Work out the finished part from the listing and answer in its coordinate system (mm). Face numbers are marked on the shaded views. Coordinates: 2 decimals unless noted, no trailing zeros. Write each loop counter-clockwise with the first axis right and the second up, starting at its lowest first coordinate (ties: lowest second). Pieces come first, ordered by that corner, then holes. Notation, with made-up numbers: M -35,-21.5 L -5,-21.5 A19 ccw -5,-16.5 Z; hole C 9,33.5 d2. An arc over 180 degrees is marked long. Use CSV: the item, a comma, the result in double quotes.
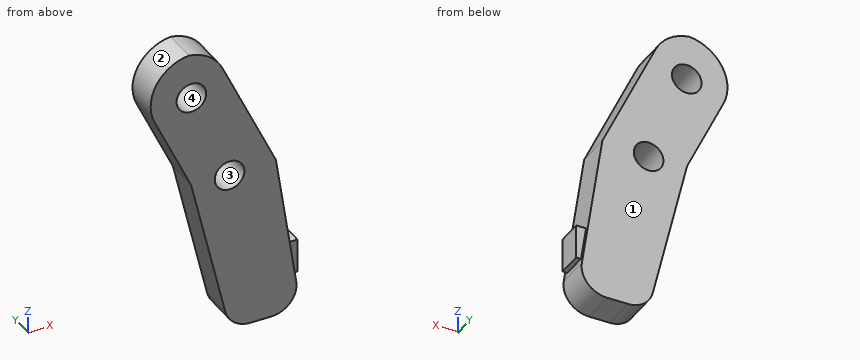
from build123d import *

# Parameters (mm, degrees)
BOSS_EXTRUDE1_DEPTH = 4
FILLET1_R           = 5
FILLET2_R           = 3
SKETCH2_R           = 1.75
CUT_EXTRUDE1_DEPTH  = 42.213228115
BOSS_EXTRUDE2_REACH = 42.084
SKETCH4_W           = 4
SKETCH4_H           = 3


with BuildPart() as part:
    # Sketch1 → Boss-Extrude1 (new body)
    with BuildSketch(Plane(origin=(0, 0, 0), x_dir=(1, 0, 0), z_dir=(0, 1, 0))):
        Polygon((0, 0), (7.627319971, 16.304109607), (12.214275277, 35.771000499), (20.559764671, 35.771000499), (17.627319971, 16.304109607), (10, 0), align=None)
    extrude(amount=BOSS_EXTRUDE1_DEPTH)

    # Fillet1
    # the kernel refuses this fillet: 5 mm, written as the material it takes off along each edge
    with BuildSketch(Plane(origin=(10, -7.952504215, 0), x_dir=(0.42373999836860227, 0, -0.9057838670359375), z_dir=(0, 1, 0))) as fillet1_piece_1:
        with BuildLine():
            CenterArc((FILLET1_R * 0.636200337192, FILLET1_R), FILLET1_R, 205.070935448, 64.929064552)
            Line((-FILLET1_R * 0.269583529844, FILLET1_R * 0.576260001631), (0, 0))
            Line((0, 0), (FILLET1_R * 0.636200337192, 0))
        make_face()
    extrude(amount=19.90500843, mode=Mode.SUBTRACT)
    with BuildSketch(Plane(origin=(0, -19.647899049, 0), x_dir=(0.42373999836860193, 0, -0.9057838670359376), z_dir=(0, 1, 0))) as fillet1_piece_2:
        with BuildLine():
            CenterArc((FILLET1_R * 1.57183192391, -FILLET1_R), FILLET1_R, 90, 115.070935448)
            Line((FILLET1_R * 0.666048056873, -FILLET1_R * 1.42373999837), (0, 0))
            Line((0, 0), (FILLET1_R * 1.57183192391, 0))
        make_face()
    extrude(amount=43.295798098, mode=Mode.SUBTRACT)

    # Fillet2
    fillet2_edges = [part.edges().sort_by_distance(p)[0] for p in [
        (12.214275277, 2, -35.771000499),
        (20.559764671, 2, -35.771000499),
    ]]
    fillet(fillet2_edges, radius=FILLET2_R)

    # Sketch2 → Cut-Extrude1 (cut, through all)
    with BuildSketch(Plane(origin=(0, 4, 0), x_dir=(1, 0, 0), z_dir=(0, 1, 0))):
        with Locations(Location((7.667711585, 5.413915862, 0), (0, 0, 270))):
            Circle(SKETCH2_R)
        with Locations(Location((12.170024678, 16.537277621, 0), (0, 0, 270))):
            Circle(SKETCH2_R)
    extrude(amount=-CUT_EXTRUDE1_DEPTH, mode=Mode.SUBTRACT)

    # Boss-Extrude2: up to this plane
    boss_extrude2_end = Plane(origin=(17.627319971, 4, -16.304109607), z_dir=(-0.9888436763539994, 0, -0.1489569861896618))
    # Sketch4 → Boss-Extrude2 (add, up to the surface)
    with BuildSketch(Plane(origin=(20.5, 0, 0), x_dir=(0, 0, -1), z_dir=(1, 0, 0)), mode=Mode.PRIVATE) as boss_extrude2_sk1:
        with Locations((29.561107497, 2.091926215)):
            Rectangle(SKETCH4_W, SKETCH4_H)
    boss_extrude2_tool1 = split(extrude(boss_extrude2_sk1.sketch, amount=-BOSS_EXTRUDE2_REACH, mode=Mode.PRIVATE), bisect_by=boss_extrude2_end, keep=Keep.BOTH, mode=Mode.PRIVATE)
    add(boss_extrude2_tool1.solids().sort_by_distance((20.5, 2.091926, -29.561107))[0])


solid = part.part
Item 1: Consider probe 1 along X at (y, z) = (1.65, -6); probe 2 along X at (y, z) = (1.85, -18); probe 3 along Z at (x, y) = (6.75, 1.6). Determine where each line is inside the solid, lowest interval first.
Answer:
probe 1,"x = 2.96 to 6.02, 9.32 to 12.81"
probe 2,"x = 8.03 to 11.21, 13.13 to 17.88"
probe 3,"z = -14.43 to -6.9, -3.92 to -0.12"
Item 2: The part is cut by section A-A (x = 7). Write down the section's boundary in (y, z), then the cut area to 3 significant figures.
Answer:
outline,"M 0,-14.96 L 4,-14.96 L 4,-7.03 L 0,-7.03 Z; M 0,-3.8 L 4,-3.8 L 4,-0.07 L 0,-0.07 Z"
area,"46.6 mm2"
Item 3: The part is cut by section B-B (y = 2.3). Write down the section's boundary in (x, z), then the cut area to 3 significant figures.
Answer:
outline,"M 3.33,-7.12 L 7.63,-16.3 L 11.67,-33.46 A3 ccw 14.59,-35.77 L 17.07,-35.77 A3 ccw 20.04,-32.32 L 19.93,-31.56 L 20.5,-31.56 L 20.5,-27.56 L 19.32,-27.56 L 17.63,-16.3 L 11.35,-2.88 A5 ccw 7.34,-0.03 A5 ccw Z; hole C 7.67,-5.41 d3.5; hole C 12.17,-16.54 d3.5"
area,"306 mm2"
Item 4: The part is cut by section C-C (z = -31). Write down the section's boundary in (x, y), then the cut area to 3 significant figures.
Answer:
outline,"M 11.09,0 L 19.84,0 L 19.84,0.59 L 20.5,0.59 L 20.5,3.59 L 19.84,3.59 L 19.84,4 L 11.09,4 Z"
area,"37.0 mm2"
Item 5: For a pull along Z with two mould halves and no side action, classify the marked faces 1, 2, 3 and 4 as released by +Z, released by -Z, zero draft, split by the parting line, or undercut.
Answer:
face 1,"zero draft"
face 2,"split by the parting line"
face 3,"undercut"
face 4,"undercut"
Item 6: The part is cut by section D-D (x = 12.5). Write down the section's boundary in (y, z).
Answer:
outline,"M 0,-34.92 L 4,-34.92 L 4,-18.26 L 0,-18.26 Z; M 0,-14.82 L 4,-14.82 L 4,-5.34 L 0,-5.34 Z"
Item 7: Given pin 1 (0.5 mm diameter, centred on x = 20, y = 2.5, fed in from -Z); pin 2 (1 mm diameter, centred on y = 3, z = -18, fed in from -X); pin 3 (3 mm diameter, centred on x = 13.5, z = -7, fed in from +Y); pin 4 (0.6 mm diameter, centred on x = 20, z = -29, fed in from -Y), each flat-ended and moving along its own axis, determine where each tip first touches the part or whether it passes through.
Answer:
pin 1,"stops at z = -34.13"
pin 2,"stops at x = 7.91"
pin 3,"stops at y = 4"
pin 4,"stops at y = 0.59"
